The listing builds one solid part. Answer for the finished solid, in the listing's coordinates (mm). Face numbers are marked on the shaded views. Round coordinates to 2 decimals unless told otherwise and drop trailing zeros. Order: outer loops, then holes, each group sorted by start corner. A loop starts at its lowest first (then second) coordinate and runs counter-clockwise, first axis right, second up. Notation, with made-up numbers: (-26, -5.5) -> (-13, -5.5) arc R14 cw to (-13, 6.5) -> close; hole circle Ø11 at (41, -29.5). An arc over 180 degrees is marked (long way). Return JSON: item names as keys, results as strings. Group by question number.
(1) The part is cut by section C-C (y = 19). Determine the outline of the cut face in (x, z), plus the area to 3 significant figures.
(2) The part is cut by section B-B (x = 0). Determine the outline of the cut face in (y, z).
(3) Each of these flat-tipped pins is pushed along its axis until it touches: pin 1 (12 mm diameter, centred on x = -8.5, z = 2, fed in from +Y); pin 2 (3 mm diameter, centred on y = 19.5, z = -13, fed in from -X); pin 3 (8 mm diameter, centred on x = -4.5, y = 9.5, fed in from -Z); pin 4 (2 mm diameter, centred on x = 7.5, z = -7, fed in from -Y). Where does it stop, or does it pass through?
(4) The part is cut by section A-A (z = 0). Determine the outline of the cut face in (x, y), plus the area to 3 significant figures.
(5) Determine the mould class of the marked faces 1, 2 and 3 for opening direction X: +X half, -X half, draft (parallel to the pull), parting line (faces both ways), or undercut.
(6) Consider line 1 (X direction, y = 23.75, z = 0); line 2 (X direction, y = 0.9, z = 0). Determine where each line is inside the solid, lowest interval first. Write a range as [from, to].
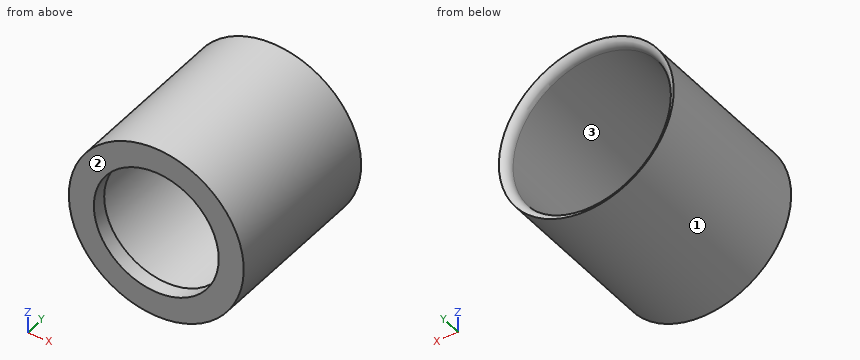
from build123d import *

# Parameters (mm, degrees)
SKETCH1_R            = 17.5
SKETCH1_R_2          = 16
BOSS_EXTRUDE1_DEPTH  = 34
SKETCH2_R            = 17.5
BOSS_EXTRUDE2_DEPTH  = 3
FILLET1_R            = 2
SKETCH3_R            = 11
BOSS_EXTRUDE3_DEPTH  = 30
CUT_EXTRUDE1_DEPTH   = 35
SKETCH6_W            = 7.99098924
SKETCH6_H            = 6.392791393
BOSS_EXTRUDE4_DEPTH  = 24
SPLIT1_OUTLINE_R     = 11
SPLIT1_DEPTH         = 33
SPLIT1_2_OUTLINE_R   = 17.5
SPLIT1_2_OUTLINE_R_2 = 11
SPLIT1_2_DEPTH       = 3
SKETCH7_R            = 17.5
SKETCH7_R_2          = 16
BOSS_EXTRUDE5_DEPTH  = 3
SKETCH8_R            = 17.5
SKETCH8_R_2          = 12.5
BOSS_EXTRUDE6_DEPTH  = 3


# Read off the part's stored shape, not the designer's step: Split1
with BuildPart() as part:
    # Sketch1 → Boss-Extrude1 (new body)
    with BuildSketch(Plane(origin=(0, 0, 0), x_dir=(1, 0, 0), z_dir=(0, 1, 0))):
        with Locations(Location((0, 0, 0), (0, 0, 270))):
            Circle(SKETCH1_R)
        with Locations(Location((0, 0, 0), (0, 0, 270))):
            Circle(SKETCH1_R_2, mode=Mode.SUBTRACT)
    extrude(amount=BOSS_EXTRUDE1_DEPTH)

    # Sketch2 → Boss-Extrude2 (add)
    with BuildSketch(Plane(origin=(0, 0, 0), x_dir=(1, 0, 0), z_dir=(0, 1, 0))):
        with Locations(Location((0, 0, 0), (0, 0, 270))):
            Circle(SKETCH2_R)
    extrude(amount=BOSS_EXTRUDE2_DEPTH)

    # Fillet1
    # the kernel refuses this fillet: 2 mm, written as the material it takes off along each edge
    with BuildSketch(Plane(origin=(0, 34, 0), x_dir=(0, 0, 1), z_dir=(-1, 0, 0))) as fillet1_piece_1:
        with BuildLine():
            CenterArc((18, -1.936491673), FILLET1_R, 104.477512186, 75.522487814)
            Line((16, -1.936491673), (15.96, -1.936491673))
            Line((15.96, -1.936491673), (15.96, 0))
            Line((15.96, 0), (16, 0.04))
            ThreePointArc((16, 0.04), (16.75, 0.04), (17.49, 0.038729833))
            Line((17.49, 0.038729833), (17.5, 0))
        make_face()
    revolve(axis=Axis((0, 34, 0), (0, 1, 0)), mode=Mode.SUBTRACT)

    # Sketch3 → Boss-Extrude3 (add)
    with BuildSketch(Plane(origin=(0, 3, 0), x_dir=(1, 0, 0), z_dir=(0, 1, 0))):
        with Locations(Location((0, 0, 0), (0, 0, 270))):
            Circle(SKETCH3_R)
    extrude(amount=BOSS_EXTRUDE3_DEPTH)

    # Sketch5 → Cut-Extrude1 (cut)
    with BuildSketch(Plane(origin=(0, 33, 0), x_dir=(1, 0, 0), z_dir=(0, 1, 0))):
        with BuildLine():
            Line((-1.077438314, 1.385334501), (1.077438314, 1.385334501))
            ThreePointArc((1.077438314, 1.385334501), (0, -1.755), (-1.077438314, 1.385334501))
        make_face()
    extrude(amount=-CUT_EXTRUDE1_DEPTH, mode=Mode.SUBTRACT)

    # Sketch6 → Boss-Extrude4 (add)
    with BuildSketch(Plane(origin=(0, 33, 0), x_dir=(1, 0, 0), z_dir=(0, 1, 0))):
        with Locations((0.014035957, -0.788514839)):
            Rectangle(SKETCH6_W, SKETCH6_H)
    extrude(amount=-BOSS_EXTRUDE4_DEPTH)

    # Split1 outline → Split1 (cut)
    with BuildSketch(Plane(origin=(0, 0, 0), x_dir=(1, 0, 0), z_dir=(0, 1, 0))):
        Circle(SPLIT1_OUTLINE_R)
    extrude(amount=SPLIT1_DEPTH, mode=Mode.SUBTRACT)

    # Split1 2 outline → Split1 2 (cut)
    with BuildSketch(Plane(origin=(0, 0, 0), x_dir=(1, 0, 0), z_dir=(0, 1, 0))):
        Circle(SPLIT1_2_OUTLINE_R)
        Circle(SPLIT1_2_OUTLINE_R_2, mode=Mode.SUBTRACT)
    extrude(amount=SPLIT1_2_DEPTH, mode=Mode.SUBTRACT)

    # Sketch7 → Boss-Extrude5 (add)
    with BuildSketch(Plane(origin=(0, 0, 0), x_dir=(-1, 0, 0), z_dir=(0, -1, 0))):
        with Locations(Location((0, 0, 0), (0, 0, 90))):
            Circle(SKETCH7_R)
        with Locations(Location((0, 0, 0), (0, 0, 90))):
            Circle(SKETCH7_R_2, mode=Mode.SUBTRACT)
    extrude(amount=-BOSS_EXTRUDE5_DEPTH)

    # Sketch8 → Boss-Extrude6 (add)
    with BuildSketch(Plane(origin=(0, 0, 0), x_dir=(-1, 0, 0), z_dir=(0, -1, 0))):
        with Locations(Location((0, 0, 0), (0, 0, 90))):
            Circle(SKETCH8_R)
        with Locations(Location((0, 0, 0), (0, 0, 90))):
            Circle(SKETCH8_R_2, mode=Mode.SUBTRACT)
    extrude(amount=-BOSS_EXTRUDE6_DEPTH)


solid = part.part
Answer below:
{
 "1": {"outline": "circle Ø35 at (0, 0); hole circle Ø32 at (0, 0)", "area": "158 mm²"},
 "2": {"outline": "(0, -17.5) -> (34, -17.5) arc R2 ccw to (32.06, -16) -> (3, -16) -> (3, -12.5) -> (0, -12.5) -> close; (0, 12.5) -> (3, 12.5) -> (3, 16) -> (32.06, 16) arc R2 ccw to (34, 17.5) -> (0, 17.5) -> close"},
 "3": {"pin 1": "stops at y = 3", "pin 2": "stops at x = -13.19", "pin 3": "stops at z = -17.49", "pin 4": "passes through"},
 "4": {"outline": "(-17.5, 0) -> (-12.5, 0) -> (-12.5, 3) -> (-16, 3) -> (-16, 32.06) arc R2 ccw to (-17.5, 34) -> close; (12.5, 0) -> (17.5, 0) -> (17.5, 34) arc R2 ccw to (16, 32.06) -> (16, 3) -> (12.5, 3) -> close", "area": "121 mm²"},
 "5": {"face 1": "parting line", "face 2": "draft", "face 3": "undercut"},
 "6": {"line 1": "x = [-17.5, -16], [16, 17.5]", "line 2": "x = [-17.5, -12.5], [12.5, 17.5]"}
}
